Part model, mm, in its own coordinate system. Face numbers are marked on the shaded views. A direction names the side the tool comes from. Give positions to 0.01 mm unless a question says otherwise; leave off trailing zeros. Order: outer loops, then holes, each group sorted by start corner. A loop starts at its lowest first (then second) coordinate and runs counter-clockwise, first axis right, second up. Notation, with made-up numbers: (27.5, -40) -> (71.5, -40) arc R25 cw to (71.5, -5) -> close; hole circle Ø2 at (-2.5, 49). An arc over 180 degrees is marked (long way). Write item = value, one per line. Start each with the question number.
(1) Probe line 1 along X through (y, z) = (0.6, -1.25); line 2 along Y through (x, z) = (-5.75, -4.5); line 3 along X through (y, z) = (3.6, -0.5). List the from-to ranges inside material, lowest first. Write a range as from..to.
(2) Two-plate mould, pull along X, no slides. Class the marked faces 1, 2, 3 and 4: pulls with the +X half, pulls with the -X half, needs draft (parallel to the pull), parting line crosses it, or undercut.
(3) Which spindle directions (+Z, -Z, +X, -X, +Y, -Y) get a long thin tool onto all of the face, cutting with end or side? Do the marked faces 5 and 6. Say none if no direction does.
(4) Saw through at D-D, the plane x = -7. List the corners of the cut face in (y, z).
(5) Flat gauge pins, fed straight in: pin 1 (1.8 mm diameter, centred on x = -7, z = 0, fed in from -Y); pin 2 (1 mm diameter, centred on x = -7.5, y = 2, fed in from +Z); pin 3 (4 mm diameter, centred on x = 0, z = 7, fed in from +Y); pin 4 (1 mm diameter, centred on x = -0.5, y = 3.5, fed in from +Z). Where does each tip first touch, or does it go through?
(6) Saw through at C-C, the plane y = 3.05. List the corners of the cut face in (x, z) (3 decimals), then the cut area to 3 significant figures.
(7) Saw through at A-A, the plane x = 0. List the corners of the cut face in (y, z) (3 decimals).
(8) Saw through at B-B, the plane z = -6. List the corners of the cut face in (x, y).
from build123d import *

# Parameters (mm, degrees)
CROQUIS1_R                        = 10
SALIENTE_EXTRUIR1_DEPTH           = 2
CROQUIS2_R                        = 4.5
SALIENTE_EXTRUIR2_DEPTH           = 2.5
DI_METRO_DE_TALADRO_3_0_3_1_D     = 3
DI_METRO_DE_TALADRO_3_0_3_1_DEPTH = 50
DI_METRO_DE_TALADRO_3_0_3_1_TIP   = 0.901290929
CROQUIS5_R                        = 3.025
CORTAR_EXTRUIR1_DEPTH             = 2.5


with BuildPart() as part:
    # Croquis1 → Saliente-Extruir1 (new body)
    with BuildSketch(Plane(origin=(0, 0, 0), x_dir=(1, 0, 0), z_dir=(0, 1, 0))):
        with Locations(Location((0, 0, 0), (0, 0, 270))):
            Circle(CROQUIS1_R)
    extrude(amount=SALIENTE_EXTRUIR1_DEPTH)

    # Croquis2 → Saliente-Extruir2 (add)
    with BuildSketch(Plane(origin=(0, 2, 0), x_dir=(1, 0, 0), z_dir=(0, 1, 0))):
        with Locations(Location((0, 0, 0), (0, 0, 270))):
            Circle(CROQUIS2_R)
    extrude(amount=SALIENTE_EXTRUIR2_DEPTH)

    # Diámetro de taladro Ø3.0 (3)1
    with Locations(Plane(origin=(0, 2, 0), x_dir=(1, 0, 0), z_dir=(0, 1, 0))):
        with Locations((0, 7), (-7, 0), (7, 0), (0, -7)):
            Hole(DI_METRO_DE_TALADRO_3_0_3_1_D / 2, depth=DI_METRO_DE_TALADRO_3_0_3_1_DEPTH)
            with Locations((0, 0, -(DI_METRO_DE_TALADRO_3_0_3_1_DEPTH + DI_METRO_DE_TALADRO_3_0_3_1_TIP / 2))):  # 118° drill point
                Cone(0, DI_METRO_DE_TALADRO_3_0_3_1_D / 2, DI_METRO_DE_TALADRO_3_0_3_1_TIP, mode=Mode.SUBTRACT)

    # Croquis5 → Cortar-Extruir1 (cut)
    with BuildSketch(Plane(origin=(0, 4.5, 0), x_dir=(1, 0, 0), z_dir=(0, 1, 0))):
        with Locations(Location((0, 0, 0), (0, 0, 270))):
            Circle(CROQUIS5_R)
    extrude(amount=-CORTAR_EXTRUIR1_DEPTH, mode=Mode.SUBTRACT)


solid = part.part
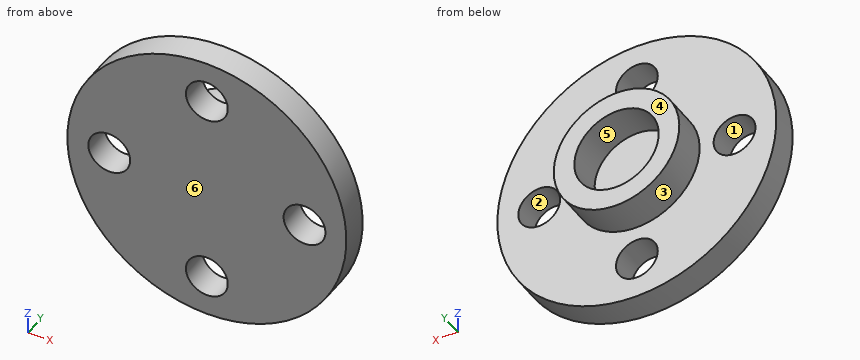
Results list:
q1.line_1 = -9.92..-7.83, -6.17..6.17, 7.83..9.92
q1.line_2 = 0..2
q1.line_3 = -4.47..-2.98, 2.98..4.47
q2.face_1 = undercut
q2.face_2 = undercut
q2.face_3 = parting line crosses it
q2.face_4 = needs draft
q3.face_5 = +Y
q3.face_6 = +Z, -Z, +X, -X, -Y
q4.outline = (0, -7.14) -> (2, -7.14) -> (2, -1.5) -> (0, -1.5) -> close; (0, 1.5) -> (2, 1.5) -> (2, 7.14) -> (0, 7.14) -> close
q5.pin_1 = through
q5.pin_2 = 7.14
q5.pin_3 = 2
q5.pin_4 = 4.5
q6.outline = circle Ø9 at (0, 0); hole circle Ø6.05 at (0, 0)
q6.area = 34.9 mm^2
q7.outline = (0, -10) -> (2, -10) -> (2, -8.5) -> (0, -8.5) -> close; (0, -5.5) -> (2, -5.5) -> (2, -4.5) -> (4.5, -4.5) -> (4.5, -3.025) -> (2, -3.025) -> (2, 3.025) -> (4.5, 3.025) -> (4.5, 4.5) -> (2, 4.5) -> (2, 5.5) -> (0, 5.5) -> close; (0, 8.5) -> (2, 8.5) -> (2, 10) -> (0, 10) -> close
q8.outline = (-8, 0) -> (-1.12, 0) -> (-1.12, 2) -> (-8, 2) -> close; (1.12, 0) -> (8, 0) -> (8, 2) -> (1.12, 2) -> close
